Read the model definition and answer for the solid it produces. Units are mm, in the model's axes. A direction names the side the tool comes from. Coordinates: 2 decimals unless noted, no trailing zeros. Write each loop counter-clockwise with the first axis right and the second up, starting at its lowest first coordinate (ties: lowest second). Pieces come first, ordered by that corner, then holes. Notation, with made-up numbers: (-15, -22) - (6, -22) arc R18 ccw to (6, 2) - close; hole circle Ø8 at (17.5, -30.75). An arc over 180 degrees is marked (long way). Return JSON: item names as keys, results as strings.
```python
from build123d import *

# Parameters (mm, degrees)
EXTRUDE_1_DEPTH          = 26
SKETCH_2_R               = 5
CUT_EXTRUDE_1_DEPTH      = 26
SKETCH_5_R               = 2.5
CUT_EXTRUDE_3_DEPTH      = 12
CUT_EXTRUDE_START        = -12
SKETCH_6_R               = 2.5
CUT_EXTRUDE_4_DEPTH      = 12
CUT_EXTRUDE_5_REACH      = 109.051
SKETCH_7_R               = 1.5
CUT_EXTRUDE_6_REACH      = 107.243
CUT_EXTRUDE_6_END_RADIUS = 20
SKETCH_8_R               = 1.5
SKETCH_10_R              = 2.5
CUT_EXTRUDE_7_DEPTH      = 12
CUT_EXTRUDE_8_REACH      = 107.243
CUT_EXTRUDE_START_2      = -26
CUT_EXTRUDE_9_DEPTH      = 26
SKETCH_13_R              = 1.5
CUT_EXTRUDE_10_DEPTH     = 5
CUT_EXTRUDE_START_3      = -5
SKETCH_14_R              = 1.5
CUT_EXTRUDE_11_DEPTH     = 5


# Read off the part's stored shape, not the designer's step: 切除-拉伸9
with BuildPart() as part:
    # 草图1 → 凸台-拉伸1 (new body)
    with BuildSketch(Plane.XY):
        with BuildLine():
            ThreePointArc((20, 0), (0, 20), (-20, 0))
            Line((-20, 0), (20, 0))
        make_face()
        with BuildLine():
            Line((20, 0), (-20, 0))
            ThreePointArc((-20, 0), (0, -20), (20, 0))
        make_face()
        with BuildLine():
            ThreePointArc((20, 0), (0, -20), (-20, 0))
            Line((-20, 0), (-20, -55))
            Line((-20, -55), (20, -55))
            Line((20, -55), (20, 0))
        make_face()
        Polygon((20, -55), (-20, -55), (-17.7, -75), (-12.2, -100), (-7.2, -100), (12.8, -75), align=None)
    extrude(amount=EXTRUDE_1_DEPTH)

    # 草图2 → 切除-拉伸1 (cut)
    with BuildSketch(Plane.XY.offset(26)):
        Circle(SKETCH_2_R)
    extrude(amount=-CUT_EXTRUDE_1_DEPTH, mode=Mode.SUBTRACT)

    # 草图5 → 切除-拉伸3 (cut)
    with BuildSketch(Plane.ZY.offset(20)):
        with Locations(Location((13, 0, 0), (0, 0, 270))):
            Circle(SKETCH_5_R)
    extrude(amount=-CUT_EXTRUDE_3_DEPTH, mode=Mode.SUBTRACT)

    # 草图6 → 切除-拉伸4 (cut)
    with BuildSketch(Plane(origin=(20, 0, 0), x_dir=(0, 0, -1), z_dir=(1, 0, 0)).offset(CUT_EXTRUDE_START)):
        with Locations(Location((-13, 0, 0), (0, 0, 270))):
            Circle(SKETCH_6_R)
    extrude(amount=CUT_EXTRUDE_4_DEPTH, mode=Mode.SUBTRACT)

    # 切除-拉伸5: up to this face of the body (flat: up to its plane)
    cut_extrude_5_end = Plane(part.part.faces().sort_by_distance((-8, 0, 13))[0])
    # 草图7 → 切除-拉伸5 (cut, up to the picked face)
    with BuildSketch(Plane(origin=(8, 0, 0), x_dir=(0, 0, -1), z_dir=(1, 0, 0)), mode=Mode.PRIVATE) as cut_extrude_5_sk1:
        with Locations(Location((-13, 0, 0), (0, 0, 90))):
            Circle(SKETCH_7_R)
    cut_extrude_5_tool1 = split(extrude(cut_extrude_5_sk1.sketch, amount=-CUT_EXTRUDE_5_REACH, mode=Mode.PRIVATE), bisect_by=cut_extrude_5_end, keep=Keep.BOTH, mode=Mode.PRIVATE)
    add(cut_extrude_5_tool1.solids().sort_by(Axis((8, 0, 13), (-1, 0, 0)))[0], mode=Mode.SUBTRACT)

    # 切除-拉伸6: up to this cylinder (the profile starts inside it)
    cut_extrude_6_end = Plane(origin=(0, 0, 13), z_dir=(0, 0, -1)) * Cylinder(CUT_EXTRUDE_6_END_RADIUS, 255.486, mode=Mode.PRIVATE)
    # 草图8 → 切除-拉伸6 (cut, up to the surface)
    with BuildSketch(Plane(origin=(0, 0, 0), x_dir=(1, 0, 0), z_dir=(0, 1, 0)), mode=Mode.PRIVATE) as cut_extrude_6_sk1:
        with Locations(Location((0, -13, 0), (0, 0, 90))):
            Circle(SKETCH_8_R)
    cut_extrude_6_tool1 = extrude(cut_extrude_6_sk1.sketch, amount=CUT_EXTRUDE_6_REACH, mode=Mode.PRIVATE) & cut_extrude_6_end
    add(cut_extrude_6_tool1.solids().sort_by_distance((0, 0, 13))[0], mode=Mode.SUBTRACT)

    # 草图10 → 切除-拉伸7 (cut)
    with BuildSketch(Plane(origin=(0, 20, 0), x_dir=(1, 0, 0), z_dir=(0, 1, 0))):
        with Locations(Location((0, -13, 0), (0, 0, 270))):
            Circle(SKETCH_10_R)
    extrude(amount=-CUT_EXTRUDE_7_DEPTH, mode=Mode.SUBTRACT)

    # 草图11 → 切除-拉伸8 (cut, up to next)
    with BuildSketch(Plane.XY.offset(26), mode=Mode.PRIVATE) as cut_extrude_8_sk1:
        Polygon((-7.5, -55), (-20, -55), (-18.275, -70), (-7.5, -70), align=None)
    cut_extrude_8_tool1 = extrude(cut_extrude_8_sk1.sketch, amount=-CUT_EXTRUDE_8_REACH, mode=Mode.PRIVATE) & part.part
    # 草图11 → 切除-拉伸8 (cut, up to next)
    with BuildSketch(Plane.XY.offset(26), mode=Mode.PRIVATE) as cut_extrude_8_sk2:
        Polygon((20, -55), (7.5, -55), (7.5, -70), (14.6, -70), align=None)
    cut_extrude_8_tool2 = extrude(cut_extrude_8_sk2.sketch, amount=-CUT_EXTRUDE_8_REACH, mode=Mode.PRIVATE) & part.part
    add(cut_extrude_8_tool1.solids().sort_by_distance((-13.329404, -62.314715, 26))[0], mode=Mode.SUBTRACT)
    add(cut_extrude_8_tool2.solids().sort_by_distance((12.52398, -61.811224, 26))[0], mode=Mode.SUBTRACT)

    # 切除-拉伸9 outline → 切除-拉伸9 (cut)
    with BuildSketch(Plane.XY.offset(26).offset(CUT_EXTRUDE_START_2)):
        with BuildLine():
            ThreePointArc((-7.5, -55), (-16.389505797, -49.97236528), (-20, -40.419106371))
            Line((-20, -40.419106371), (-20, -55))
            Line((-20, -55), (-7.5, -55))
        make_face()
        with BuildLine():
            ThreePointArc((20, -40.419106371), (16.389505797, -49.97236528), (7.5, -55))
            Line((7.5, -55), (20, -55))
            Line((20, -55), (20, -40.419106371))
        make_face()
    extrude(amount=CUT_EXTRUDE_9_DEPTH, mode=Mode.SUBTRACT)

    # 草图13 → 切除-拉伸10 (cut)
    with BuildSketch(Plane.XY.offset(26)):
        with Locations((-12.5, -27.5)):
            Circle(SKETCH_13_R)
        with Locations((12.5, -27.5)):
            Circle(SKETCH_13_R)
        with Locations((12.5, 0)):
            Circle(SKETCH_13_R)
        with Locations((0, 12.5)):
            Circle(SKETCH_13_R)
        with Locations((-12.5, 0)):
            Circle(SKETCH_13_R)
        with Locations((-9.7, -87.5)):
            Circle(SKETCH_13_R)
    extrude(amount=-CUT_EXTRUDE_10_DEPTH, mode=Mode.SUBTRACT)

    # 草图14 → 切除-拉伸11 (cut)
    with BuildSketch(Plane(origin=(0, 0, 0), x_dir=(-1, 0, 0), z_dir=(0, 0, -1)).offset(CUT_EXTRUDE_START_3)):
        with Locations(Location((12.5, 0, 0), (0, 0, 180))):
            Circle(SKETCH_14_R)
        with Locations(Location((0, 12.5, 0), (0, 0, 180))):
            Circle(SKETCH_14_R)
        with Locations(Location((-12.5, 0, 0), (0, 0, 180))):
            Circle(SKETCH_14_R)
        with Locations(Location((-12.5, -27.5, 0), (0, 0, 180))):
            Circle(SKETCH_14_R)
        with Locations(Location((12.5, -27.5, 0), (0, 0, 180))):
            Circle(SKETCH_14_R)
        with Locations(Location((9.7, -87.5, 0), (0, 0, 180))):
            Circle(SKETCH_14_R)
    extrude(amount=CUT_EXTRUDE_11_DEPTH, mode=Mode.SUBTRACT)


solid = part.part
```
(1) A cutting plane is placed at B-B (z = 18.75). Determine the outline of the cut face in (x, y) (3 decimals), and give its area (3 significant figures).
Answer:
{"outline": "(-20, -40.419) arc R15 ccw to (-7.5, -55) - (-7.5, -70) - (-18.275, -70) - (-17.7, -75) - (-12.2, -100) - (-7.2, -100) - (12.8, -75) - (14.6, -70) - (7.5, -70) - (7.5, -55) arc R15 ccw to (20, -40.419) - (20, 0) arc R20 ccw to (-20, 0) - close; hole circle Ø10 at (0, 0)", "area": "3,490 mm²"}
(2) A cutting plane is placed at C-C (x = -9.7). Determine the outline of the cut face in (y, z).
Answer:
{"outline": "(-100, 0) - (-89, 0) - (-89, 5) - (-86, 5) - (-86, 0) - (-70, 0) - (-70, 26) - (-86, 26) - (-86, 21) - (-89, 21) - (-89, 26) - (-100, 26) - close; (-54.45, 0) - (17.49, 0) - (17.49, 26) - (-54.45, 26) - close; hole circle Ø5 at (0, 13)"}
(3) Which of the six approach directions +Z, -Z, +X, -X, +Y, -Y give full straight-line access (tool end or side, diameter ignored) to faces 1 (the face through (8, 0, 15)), 2 (the face through (12, -28, 5)), 3 (the face through (12, -27, 21)), 4 (the face through (16.484, -49.861, 12.818))?
Answer:
{"face 1": "+X", "face 2": "-Z", "face 3": "+Z", "face 4": "+Z, -Z, +X"}
(4) A cutting plane is placed at D-D (y = -66). Determine the outline of the cut face in (x, z), and give its area (3 significant figures).
Answer:
{"outline": "(-7.5, 0) - (7.5, 0) - (7.5, 26) - (-7.5, 26) - close", "area": "390 mm²"}
(5) Straight lines are drawn through the part: line 1 (Y direction, x = -9.7, z = 1.2); line 2 (Y direction, x = 0.5, z = 3) (3 decimals); line 3 (X direction, y = 11, z = 13). For each, find the intervals that lie inside material, in ascending order. Write a range as from..to.
Answer:
{"line 1": "-100..-89, -86..-70, -54.45..17.49", "line 2": "-90.375..-4.975, 4.975..11.086, 13.914..19.994", "line 3": "-16.7..-2.5, 2.5..16.7"}
(6) Determine the mould class of faces 5 (the face through (0, 20, 10)), 6 (the face through (-12.695, -28.987, 2.535)), 7 (the face through (20, -20, 13)) for opening direction X: +X half, -X half, draft (parallel to the pull), parting line (faces both ways), or undercut.
Answer:
{"face 5": "parting line", "face 6": "undercut", "face 7": "+X half"}
(7) Flat-ended cylindrical pins translate along their axes: P1, Ø8, axis at y = -84, z = 7, coming from the +X side; P2, Ø1.5, axis at x = 0, y = 12.5, coming from the -Z side; P3, Ø4.5, axis at y = -62, z = 8.5, coming from the -X side. Find the tip coordinate at first contact, or state that the pin passes through.
Answer:
{"P1": "x = 8.8", "P2": "z = 5", "P3": "x = -7.5"}
(8) A cutting plane is placed at A-A (y = -27.5). Determine the outline of the cut face in (x, z).
Answer:
{"outline": "(-20, 0) - (-14, 0) - (-14, 5) - (-11, 5) - (-11, 0) - (11, 0) - (11, 5) - (14, 5) - (14, 0) - (20, 0) - (20, 26) - (14, 26) - (14, 21) - (11, 21) - (11, 26) - (-11, 26) - (-11, 21) - (-14, 21) - (-14, 26) - (-20, 26) - close"}
